from build123d import *

# Parameters (mm, degrees)
BOSS_EXTRUDE1_DEPTH          = 4
BOSS_EXTRUDE2_DEPTH          = 3
BOSS_EXTRUDE3_DEPTH          = 3
CUT_EXTRUDE1_DEPTH           = 2
F_5_0_5_DIAMETER_HOLE1_D     = 5
F_5_0_5_DIAMETER_HOLE1_DEPTH = 11.5
SKETCH7_W                    = 2
SKETCH7_H                    = 21.25889
M20_CLEARANCE_HOLE1_D        = 23.618330199
M20_CLEARANCE_HOLE1_DEPTH    = 4
F_4_0_4_DIAMETER_HOLE2_D     = 4
F_4_0_4_DIAMETER_HOLE2_DEPTH = 27.25889
FILLET1_R                    = 2


with BuildPart() as part:
    # Sketch1 → Boss-Extrude1 (new body)
    with BuildSketch(Plane(origin=(0, 5.770898059, 0), x_dir=(1, 0, 0), z_dir=(0, 1, 0))):
        with BuildLine():
            Line((7, -23.75889), (7, 4.24111))
            ThreePointArc((7, 4.24111), (10.353454391, 15.21648372), (1.438437052, 7.989662117))
            ThreePointArc((1.438437052, 7.989662117), (-15.414893863, -11.667157982), (1.252670952, -31.481739039))
            ThreePointArc((1.252670952, -31.481739039), (11.8133717, -33.340991741), (7, -23.75889))
        make_face()
    extrude(amount=-BOSS_EXTRUDE1_DEPTH)

    # Sketch2 → Boss-Extrude2 (add)
    with BuildSketch(Plane.XY.offset(17.5)):
        with BuildLine():
            Line((-4.913051605, -1.660534859), (-4.913051605, 1.770898059))
            Line((-4.913051605, 1.770898059), (-12.913051605, 1.770898059))
            Line((-12.913051605, 1.770898059), (-12.913051605, -1.660534859))
            ThreePointArc((-12.913051605, -1.660534859), (-8.913051605, -5.660534859), (-4.913051605, -1.660534859))
        make_face()
    extrude(amount=-BOSS_EXTRUDE2_DEPTH)

    # Sketch3 → Boss-Extrude3 (add)
    with BuildSketch(Plane.XY.offset(9.5)):
        with BuildLine():
            Line((-4.913051605, -1.729101941), (-4.913051605, 0.01125604))
            Line((-4.913051605, 0.01125604), (-5.962229818, 1.770898059))
            Line((-5.962229818, 1.770898059), (-12.913051605, 1.770898059))
            Line((-12.913051605, 1.770898059), (-12.913051605, -1.729101941))
            ThreePointArc((-12.913051605, -1.729101941), (-8.913051605, -5.729101941), (-4.913051605, -1.729101941))
        make_face()
    extrude(amount=-BOSS_EXTRUDE3_DEPTH)

    # Sketch4 → Cut-Extrude1 (cut)
    with BuildSketch(Plane(origin=(0, 0, 6.5), x_dir=(-1, 0, 0), z_dir=(0, 0, -1))):
        Polygon((7.253169581, 1.145898059), (5.593287557, -1.729101941), (7.253169581, -4.604101941), (10.572933629, -4.604101941), (12.232815653, -1.729101941), (10.572933629, 1.145898059), align=None)
    extrude(amount=-CUT_EXTRUDE1_DEPTH, mode=Mode.SUBTRACT)

    # Ø5.0 (5) Diameter Hole1
    with Locations(Plane(origin=(0, 5.770898059, 0), x_dir=(1, 0, 0), z_dir=(0, 1, 0))):
        with Locations((7, -29.75889), (7, 10.24111)):
            Hole(F_5_0_5_DIAMETER_HOLE1_D / 2, depth=F_5_0_5_DIAMETER_HOLE1_DEPTH)

    # Sketch7 → Ø4.0 (4) Diameter Hole1 (revolve, cut)
    with BuildSketch(Plane(origin=(-8.913051605, -1.729101941, 14.5), x_dir=(0, 1, 0), z_dir=(1, 0, 0))):
        with Locations((1, 10.629445)):
            Rectangle(SKETCH7_W, SKETCH7_H)
    revolve(axis=Axis((-8.913051605, -1.729101941, 8.15), (0, 0, 1)), mode=Mode.SUBTRACT)

    # M20 Clearance Hole1
    with Locations(Plane(origin=(0, 5.770898059, 0), x_dir=(1, 0, 0), z_dir=(0, 1, 0))):
        with Locations((5.844097137, -9.75889)):
            Hole(M20_CLEARANCE_HOLE1_D / 2, depth=M20_CLEARANCE_HOLE1_DEPTH)

    # Ø4.0 (4) Diameter Hole2
    with Locations(Plane(origin=(0, 0, 8.5), x_dir=(-1, 0, 0), z_dir=(0, 0, -1))):
        with Locations((8.913051605, -1.729101941)):
            Hole(F_4_0_4_DIAMETER_HOLE2_D / 2, depth=F_4_0_4_DIAMETER_HOLE2_DEPTH)

    # Fillet1
    fillet1_edges = [part.edges().sort_by_distance(p)[0] for p in [
        (1.438437052, 3.770898059, -7.989662117),
        (1.252670952, 3.770898059, 31.481739039),
        (7, 3.770898059, -1.993567995),
        (7, 3.770898059, 21.511347995),
    ]]
    fillet(fillet1_edges, radius=FILLET1_R)


solid = part.part
The model under review builds one solid part; all positions refer to its coordinate system, in mm. A direction names the side the tool comes from. Round coordinates to 2 decimals unless told otherwise and drop trailing zeros. Loops run counter-clockwise (first coordinate to the right, second up) from the corner with the lowest first, then second, coordinate; pieces in that order, holes last. Notation, with made-up numbers: (-34.5, 27) -> (-9.5, 27) arc R4 cw to (-9.5, 31) -> close; hole circle Ø5 at (-5.75, 15.25). An arc over 180 degrees is marked (long way). Write item = value, one per line. Start each with the question number.
Item 1: Insertion check: pin 1 (1.4 mm diameter, centred on y = -0.5, z = 7.5, fed in from +X); pin 2 (2.5 mm diameter, centred on x = -8.91, y = -1.73, fed in from -Z); pin 3 (6 mm diameter, centred on x = -4, z = 27.5, fed in from -Y); pin 4 (3.5 mm diameter, centred on y = 0.5, z = 8, fed in from -X). Each pin has a flat end and moves straight along its axis. Give the tip position at first contact, or say it passes through.
Item 2: Mouldability with a two-part tool opening along Z and no side actions: class faces 1 (the flat face through (-9, -4.604, 7)), 2 (the cylindrical face through (6.471, 3.743, 22.187)) as released by +Z, released by -Z, zero draft, split by the parting line, or undercut.
Item 3: Take a section at C-C on z = -6.5. Give the boundary of the cut face in (x, y).
Item 4: Take a section at A-A on x = 6.25. Give the boundary of the cut face in (y, z).
Item 5: Take a section at B-B on x = 10.25. Give the boundary of the cut face in (y, z), plus the area to 3 significant figures.
Item 6: Take a section at D-D on x = -3.75. Give the boundary of the cut face in (y, z), plus the area to 3 significant figures.
Item 7: For faces 3 (the cylindrical face through (-9, -5.66, 16.02)), 4 (the flat face through (-11, -3, 14.5)), 5 (the flat face through (-12.913, 0, 16)), 6 (the flat face through (-4.913, 0, 16)), 7 (the flat face through (-6.435, -0.271, 7.486)), list the 3-axis set-ups (+Z, -Z, +X, -X, +Y, -Y) from which the entire face can be reached by the end or side of a thin tool; tool diameter is ignored.
Item 8: To check wall thickness, follow L1, parallel to Z at x = 9.25, y = 3; L2, parallel to Z at x = 5.75, y = 2; L3, parallel to Z at x = -10.5, y = -3.5. State the ranges of each line that lie inside material, in increasing order.
Result:
q1.pin_1 = -4.91
q1.pin_2 = through
q1.pin_3 = 1.77
q1.pin_4 = -15.25
q2.face_1 = zero draft
q2.face_2 = undercut
q3.outline = (-3.57, 1.77) -> (11.69, 1.77) -> (11.69, 5.77) -> (-3.57, 5.77) -> close
q4.outline = (1.77, -16.19) -> (5.77, -16.19) -> (5.77, -12.63) -> (1.77, -12.63) -> close; (1.77, -7.86) -> (5.77, -7.86) -> (5.77, -2.46) -> (1.77, -2.46) -> close; (1.77, 21.98) -> (5.77, 21.98) -> (5.77, 27.37) -> (1.77, 27.37) -> close; (1.77, 32.14) -> (5.77, 32.14) -> (5.77, 35.71) -> (1.77, 35.71) -> close
q5.outline = (1.77, -15.28) -> (5.77, -15.28) -> (5.77, -5.2) -> (1.77, -5.2) -> close; (1.77, 24.72) -> (5.77, 24.72) -> (5.77, 34.8) -> (1.77, 34.8) -> close
q5.area = 80.7 mm²
q6.outline = (1.77, -6.42) -> (5.77, -6.42) -> (5.77, 2.87) -> (1.77, 2.87) -> close; (1.77, 16.64) -> (5.77, 16.64) -> (5.77, 29.94) -> (1.77, 29.94) -> close
q6.area = 90.4 mm²
q7.face_3 = +Z, -Y
q7.face_4 = +X, -X, -Y
q7.face_5 = +Z, -Z, -X, -Y
q7.face_6 = +Z, -Z, +X, -Y
q7.face_7 = -Z
q8.L1 = -15.8 to -11.33, -9.15 to -4.68, 24.2 to 28.67, 30.85 to 35.32
q8.L2 = -16.11 to -12.41, -8.08 to -2.17, 21.69 to 27.59, 31.92 to 35.63
q8.L3 = 8.5 to 9.5, 14.5 to 17.5
